For this review, take the finished solid that the model builds, in its own axes (mm). Round coordinates to 2 decimals unless told otherwise and drop trailing zeros. Write each loop counter-clockwise with the first axis right and the second up, starting at its lowest first coordinate (ties: lowest second). Pieces come first, ordered by that corner, then holes. Notation, with made-up numbers: (21, 61) -> (38, 61) arc R23 cw to (38, 69) -> close; hole circle Ø1 at (87.5, -0.75). An arc over 180 degrees is marked (long way). Write each question's results on one line, items separated by ' | '. Start each with the question number.
Item 1: Add section B-B (x = 3.5). State the section outline as (y, z) points, plus the area to 3 significant figures.
Item 2: Add section D-D (y = 14). State the section outline as (x, z) points.
Item 3: Add section C-C (y = -1.5). State the section outline as (x, z) points, plus the area to 3 significant figures.
Item 4: Clearance check with flat-ended pins moving along their axes: pin 1 (1 mm diameter, centred on y = -12.5, z = 4.5, fed in from +X); pin 2 (1 mm diameter, centred on x = 8.5, z = 3.5, fed in from -Y); pin 3 (2 mm diameter, centred on x = -9.5, z = 2.5, fed in from -Y); pin 4 (8 mm diameter, centred on x = -17.5, y = 3, fed in from +Z). State where each tip first meets the part, or that it passes through.
Item 5: Add section A-A (z = 2.25). State the section outline as (x, y) points (3 decimals), plus the area to 3 significant figures.
Item 6: To check wall thickness, follow line 1 along X through (y, z) = (26, 5); line 2 along X through (y, z) = (-5, 4.5); line 3 along X through (y, z) = (-9.5, 3.5). State the ranges of each line that lie inside material, in increasing order.
from build123d import *

# Parameters (mm, degrees)
F1_DEPTH = 6.9342


with BuildPart() as f1:
    # F0 (on Top) → F1 (new body)
    with BuildSketch(Plane.XY):
        with BuildLine():
            ThreePointArc((10.978713393, 0.9937852859), (11.0123726308, 0.4973992365), (11.0236, 0))
            ThreePointArc((11.0236, 0), (10.6479799387, -2.8531176256), (9.5467176412, -5.5118))
            ThreePointArc((9.5467176412, -5.5118), (7.4352089911, -8.1386377373), (4.628713393, -10.0047373422))
            Line((4.628713393, -10.0047373422), (11.7777531012, -14.1322373422))
            ThreePointArc((11.7777531012, -14.1322373422), (12.0895321135, -6.9798946201), (18.1277531012, -3.1337147141))
            Line((18.1277531012, -3.1337147141), (10.978713393, 0.9937852859))
        make_face()
        with BuildLine():
            ThreePointArc((6.35, 9.0109520562), (9.5467176412, 5.5118), (10.978713393, 0.9937852859))
            Line((10.978713393, 0.9937852859), (18.1277531012, -3.1337147141))
            ThreePointArc((18.1277531012, -3.1337147141), (19.1741700395, -3.1132418489), (20.2138057566, -3.2339278992))
            ThreePointArc((20.2138057566, -3.2339278992), (12.0108278998, 6.9344547212), (7.3062391636, 19.1226332419))
            ThreePointArc((7.3062391636, 19.1226332419), (6.8909384905, 18.1619392751), (6.35, 17.2659520562))
            Line((6.35, 17.2659520562), (6.35, 9.0109520562))
        make_face()
        with BuildLine():
            ThreePointArc((0, 11.0236), (3.3306625371, 10.5083987374), (6.35, 9.0109520562))
            Line((6.35, 9.0109520562), (6.35, 17.2659520562))
            ThreePointArc((6.35, 17.2659520562), (0, 13.9597892403), (-6.35, 17.2659520562))
            Line((-6.35, 17.2659520562), (-6.35, 9.0109520562))
            ThreePointArc((-6.35, 9.0109520562), (-3.3306625371, 10.5083987374), (0, 11.0236))
        make_face()
        with BuildLine():
            ThreePointArc((20.2138057566, -3.2339278992), (19.1741700395, -3.1132418489), (18.1277531012, -3.1337147141))
            Line((18.1277531012, -3.1337147141), (25.8267189409, -7.5787147141))
            ThreePointArc((25.8267189409, -7.5787147141), (25.8095339268, -7.5421240909), (25.7921583133, -7.5056235914))
            ThreePointArc((25.7921583133, -7.5056235914), (22.9140380361, -5.4859265713), (20.2138057566, -3.2339278992))
        make_face()
        with BuildLine():
            Line((25.8267189409, -7.5787147141), (18.1277531012, -3.1337147141))
            ThreePointArc((18.1277531012, -3.1337147141), (12.0895321135, -6.9798946201), (11.7777531012, -14.1322373422))
            Line((11.7777531012, -14.1322373422), (19.4767189409, -18.5772373422))
            ThreePointArc((19.4767189409, -18.5772373422), (20.8083845795, -18.3425243759), (22.0789973351, -17.8799589479))
            Line((22.0789973351, -17.8799589479), (26.5239973351, -10.1809931083))
            ThreePointArc((26.5239973351, -10.1809931083), (26.2892843688, -8.8493274697), (25.8267189409, -7.5787147141))
        make_face()
        with BuildLine():
            Line((11.7777531012, -14.1322373422), (4.628713393, -10.0047373422))
            ThreePointArc((4.628713393, -10.0047373422), (0, -11.0236), (-4.628713393, -10.0047373422))
            Line((-4.628713393, -10.0047373422), (-11.7777531012, -14.1322373422))
            ThreePointArc((-11.7777531012, -14.1322373422), (-12.283231549, -15.0486974262), (-12.907566593, -15.8887053427))
            ThreePointArc((-12.907566593, -15.8887053427), (0, -13.8689094423), (12.907566593, -15.8887053427))
            ThreePointArc((12.907566593, -15.8887053427), (12.283231549, -15.0486974262), (11.7777531012, -14.1322373422))
        make_face()
        with BuildLine():
            ThreePointArc((-6.35, 17.2659520562), (0, 13.9597892403), (6.35, 17.2659520562))
            Line((6.35, 17.2659520562), (6.35, 26.1559520562))
            ThreePointArc((6.35, 26.1559520562), (5.4808997893, 27.1918518455), (4.445, 28.0609520562))
            Line((4.445, 28.0609520562), (-4.445, 28.0609520562))
            ThreePointArc((-4.445, 28.0609520562), (-5.4808997893, 27.1918518455), (-6.35, 26.1559520562))
            Line((-6.35, 26.1559520562), (-6.35, 17.2659520562))
        make_face()
        with BuildLine():
            Line((6.35, 26.1559520562), (6.35, 17.2659520562))
            ThreePointArc((6.35, 17.2659520562), (6.8909384905, 18.1619392751), (7.3062391636, 19.1226332419))
            ThreePointArc((7.3062391636, 19.1226332419), (6.706067244, 22.5871023282), (6.3960184553, 26.0894761135))
            ThreePointArc((6.3960184553, 26.0894761135), (6.3730959022, 26.1227740859), (6.35, 26.1559520562))
        make_face()
        with BuildLine():
            Line((19.4767189409, -18.5772373422), (11.7777531012, -14.1322373422))
            ThreePointArc((11.7777531012, -14.1322373422), (12.283231549, -15.0486974262), (12.907566593, -15.8887053427))
            ThreePointArc((12.907566593, -15.8887053427), (16.2079707921, -17.1011757569), (19.3961398581, -18.5838525221))
            ThreePointArc((19.3961398581, -18.5838525221), (19.4364380247, -18.580649995), (19.4767189409, -18.5772373422))
        make_face()
        with BuildLine():
            Line((-11.7777531012, -14.1322373422), (-4.628713393, -10.0047373422))
            ThreePointArc((-4.628713393, -10.0047373422), (-7.4352089911, -8.1386377373), (-9.5467176412, -5.5118))
            ThreePointArc((-9.5467176412, -5.5118), (-10.7658715282, -2.3697610001), (-10.978713393, 0.9937852859))
            Line((-10.978713393, 0.9937852859), (-18.1277531012, -3.1337147141))
            ThreePointArc((-18.1277531012, -3.1337147141), (-12.0895321135, -6.9798946201), (-11.7777531012, -14.1322373422))
        make_face()
        with BuildLine():
            ThreePointArc((-10.978713393, 0.9937852859), (-9.5467176412, 5.5118), (-6.35, 9.0109520562))
            Line((-6.35, 9.0109520562), (-6.35, 17.2659520562))
            ThreePointArc((-6.35, 17.2659520562), (-6.8909384905, 18.1619392751), (-7.3062391636, 19.1226332419))
            ThreePointArc((-7.3062391636, 19.1226332419), (-12.0108278998, 6.9344547212), (-20.2138057566, -3.2339278992))
            ThreePointArc((-20.2138057566, -3.2339278992), (-19.1741700395, -3.1132418489), (-18.1277531012, -3.1337147141))
            Line((-18.1277531012, -3.1337147141), (-10.978713393, 0.9937852859))
        make_face()
        with BuildLine():
            ThreePointArc((-7.3062391636, 19.1226332419), (-6.8909384905, 18.1619392751), (-6.35, 17.2659520562))
            Line((-6.35, 17.2659520562), (-6.35, 26.1559520562))
            ThreePointArc((-6.35, 26.1559520562), (-6.3730959022, 26.1227740859), (-6.3960184553, 26.0894761135))
            ThreePointArc((-6.3960184553, 26.0894761135), (-6.706067244, 22.5871023282), (-7.3062391636, 19.1226332419))
        make_face()
        with BuildLine():
            ThreePointArc((22.0789973351, -17.8799589479), (25.5149399286, -14.7310574361), (26.5239973351, -10.1809931083))
            Line((26.5239973351, -10.1809931083), (22.0789973351, -17.8799589479))
        make_face()
        with BuildLine():
            ThreePointArc((-12.907566593, -15.8887053427), (-12.283231549, -15.0486974262), (-11.7777531012, -14.1322373422))
            Line((-11.7777531012, -14.1322373422), (-19.4767189409, -18.5772373422))
            ThreePointArc((-19.4767189409, -18.5772373422), (-19.4364380247, -18.580649995), (-19.3961398581, -18.5838525221))
            ThreePointArc((-19.3961398581, -18.5838525221), (-16.2079707921, -17.1011757569), (-12.907566593, -15.8887053427))
        make_face()
        with BuildLine():
            Line((-19.4767189409, -18.5772373422), (-11.7777531012, -14.1322373422))
            ThreePointArc((-11.7777531012, -14.1322373422), (-12.0895321135, -6.9798946201), (-18.1277531012, -3.1337147141))
            Line((-18.1277531012, -3.1337147141), (-25.8267189409, -7.5787147141))
            ThreePointArc((-25.8267189409, -7.5787147141), (-26.2892843688, -8.8493274697), (-26.5239973351, -10.1809931083))
            Line((-26.5239973351, -10.1809931083), (-22.0789973351, -17.8799589479))
            ThreePointArc((-22.0789973351, -17.8799589479), (-20.8083845795, -18.3425243759), (-19.4767189409, -18.5772373422))
        make_face()
        with BuildLine():
            Line((-4.445, 28.0609520562), (4.445, 28.0609520562))
            ThreePointArc((4.445, 28.0609520562), (0, 29.4621148722), (-4.445, 28.0609520562))
        make_face()
        with BuildLine():
            Line((-25.8267189409, -7.5787147141), (-18.1277531012, -3.1337147141))
            ThreePointArc((-18.1277531012, -3.1337147141), (-19.1741700395, -3.1132418489), (-20.2138057566, -3.2339278992))
            ThreePointArc((-20.2138057566, -3.2339278992), (-22.9140380361, -5.4859265713), (-25.7921583133, -7.5056235914))
            ThreePointArc((-25.7921583133, -7.5056235914), (-25.8095339268, -7.5421240909), (-25.8267189409, -7.5787147141))
        make_face()
        with BuildLine():
            ThreePointArc((-26.5239973351, -10.1809931083), (-25.5149399286, -14.7310574361), (-22.0789973351, -17.8799589479))
            Line((-22.0789973351, -17.8799589479), (-26.5239973351, -10.1809931083))
        make_face()
    extrude(amount=F1_DEPTH)


solid = f1.part
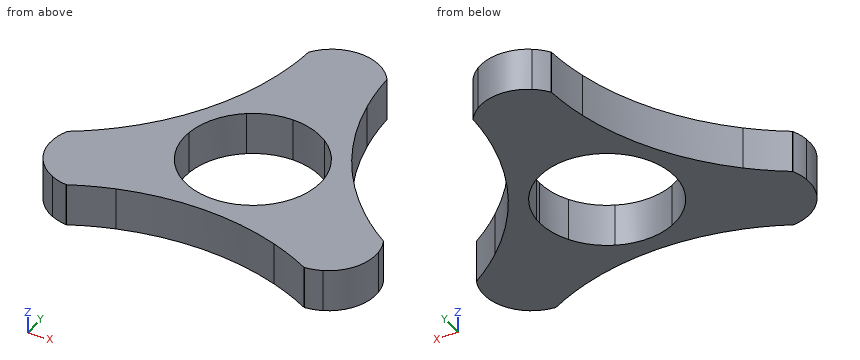
Responses:
1) outline: (-14.01, 0) -> (-10.45, 0) -> (-10.45, 6.93) -> (-14.01, 6.93) -> close; (10.45, 0) -> (28.63, 0) -> (28.63, 6.93) -> (10.45, 6.93) -> close | area: 151 mm^2
2) outline: (-8.76, 0) -> (8.76, 0) -> (8.76, 6.93) -> (-8.76, 6.93) -> close
3) outline: (-18.41, 0) -> (-10.92, 0) -> (-10.92, 6.93) -> (-18.41, 6.93) -> close; (10.92, 0) -> (18.41, 0) -> (18.41, 6.93) -> (10.92, 6.93) -> close | area: 104 mm^2
4) pin 1: stops at x = 26.47 | pin 2: stops at y = -14.84 | pin 3: stops at y = -15.19 | pin 4: stops at z = 6.93
5) outline: (-25.792, -7.506) arc R7.751 ccw to (-19.477, -18.577) arc R7.751 ccw to (-19.396, -18.584) arc R42.253 cw to (19.396, -18.584) arc R7.751 ccw to (19.477, -18.577) arc R7.751 ccw to (25.792, -7.506) arc R42.253 cw to (6.396, 26.089) arc R7.751 ccw to (-6.396, 26.089) arc R42.253 cw to start; hole circle Ø22.047 at (0, 0) | area: 921 mm^2
6) line 1: x = -6.4 to 6.4 | line 2: x = -22.29 to -9.82, 9.82 to 22.29 | line 3: x = -26.43 to -5.59, 5.59 to 26.43
